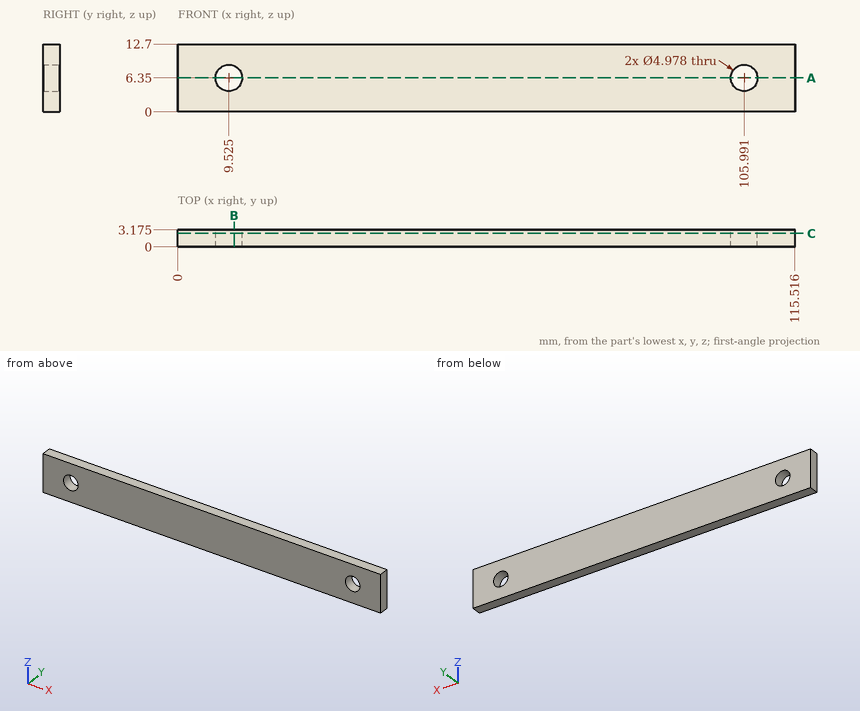
Verification items for this drawing (mm, ordinates from the low corner). Round coordinates to 2 decimals unless told otherwise and drop trailing zeros. Loops run counter-clockwise (first coordinate to the right, second up) from the corner with the lowest first, then second, coordinate; pieces in that order, holes last. Notation, with made-up numbers: (-24, 70) - (30, 70) arc R30 ccw to (30, 98) - close; hole circle Ø2 at (-0.75, 75.25). An arc over 180 degrees is marked (long way). Answer as CSV lines item,"result". Start each with the question number.
Item 1: Section check C-C (y = 2.5). Count the separate pieces of the cut face and the enclosed holes in it, and give its area (3 significant figures).
Item 2: Scan lines: line 1 (X direction, y = 2.45, z = 6.35) (1 decimal); line 2 (X direction, y = 0.3, z = 5) (1 decimal); line 3 (Z direction, x = 108, y = 2.35). Record each from-to range of solid material in increasing order. Write a range as [from, to].
Item 3: Section check A-A (z = 6.35). Record the boundary of the cut face in (x, y) (1 decimal), and give its area (3 significant figures).
Item 4: Section check B-B (x = 10.5). Record the boundary of the cut face in (y, z) (1 decimal), and give its area (3 significant figures).
Item 5: Depth check by flat-ended pin: P1, Ø5.5, axis at x = 9.525, z = 6.35, coming from the +Y side (3 decimals). Enter the tip coordinate at first touch or a pass-through.
Report:
1,separate pieces,"1"
1,enclosed holes,"2"
1,area,"1,430 mm2"
2,line 1,"x = [0, 7], [12, 103.5], [108.5, 115.5]"
2,line 2,"x = [0, 7.4], [11.6, 103.9], [108.1, 115.5]"
2,line 3,"z = [0, 4.88], [7.82, 12.7]"
3,outline,"(0, 0) - (7, 0) - (7, 3.2) - (0, 3.2) - close; (12, 0) - (103.5, 0) - (103.5, 3.2) - (12, 3.2) - close; (108.5, 0) - (115.5, 0) - (115.5, 3.2) - (108.5, 3.2) - close"
3,area,"335 mm2"
4,outline,"(0, 0) - (3.2, 0) - (3.2, 4.1) - (0, 4.1) - close; (0, 8.6) - (3.2, 8.6) - (3.2, 12.7) - (0, 12.7) - close"
4,area,"25.8 mm2"
5,P1,"stops at y = 3.175"
